Can you work these out from the drawing? Everything is in mm from the part's minimum corner. Coordinates: 2 decimals unless noted, no trailing zeros. Write each loop counter-clockwise with the first axis right and the second up, starting at its lowest first coordinate (ties: lowest second). Pieces come first, ordered by that corner, then holes. Notation, with made-up numbers: (80, 76) -> (90, 76) arc R10 cw to (90, 86) -> close; hole circle Ø1 at (41, 20.5). An arc over 180 degrees is marked (long way). Use a Markdown table: item, result. Add a question column.
Item 1: If we mould it in two halves opening along X, with no side actions, what happens to the marked faces 1 and 2? For each: pulls with the +X half, pulls with the -X half, needs draft (parallel to the pull), parting line crosses it, or undercut.
Item 2: Imagine slicing it at C-C, the plane y = 6.75. Count the separate pieces of the cut face and the enclosed holes in it, and give its area (3 significant figures).
Item 3: Imagine slicing it at B-B, the plane x = 120. Write out the boundary of the cut face in (y, z) (1 decimal).
Item 4: Imagine slicing it at D-D, the plane z = 79. Write out the boundary of the cut face in (x, y) (1 decimal).
Item 5: Imagine slicing it at A-A, the plane z = 15. Write out the boundary of the cut face in (x, y) (1 decimal).
Item 6: If I drill on line 1 along X through (y, z) = (2.25, 79) (1 decimal); line 2 along X through (y, z) = (4, 13.5); line 3 along X through (y, z) = (5.5, 59), over which ranges is the centre line in solid material (lowest first)? Write a range as from..to.
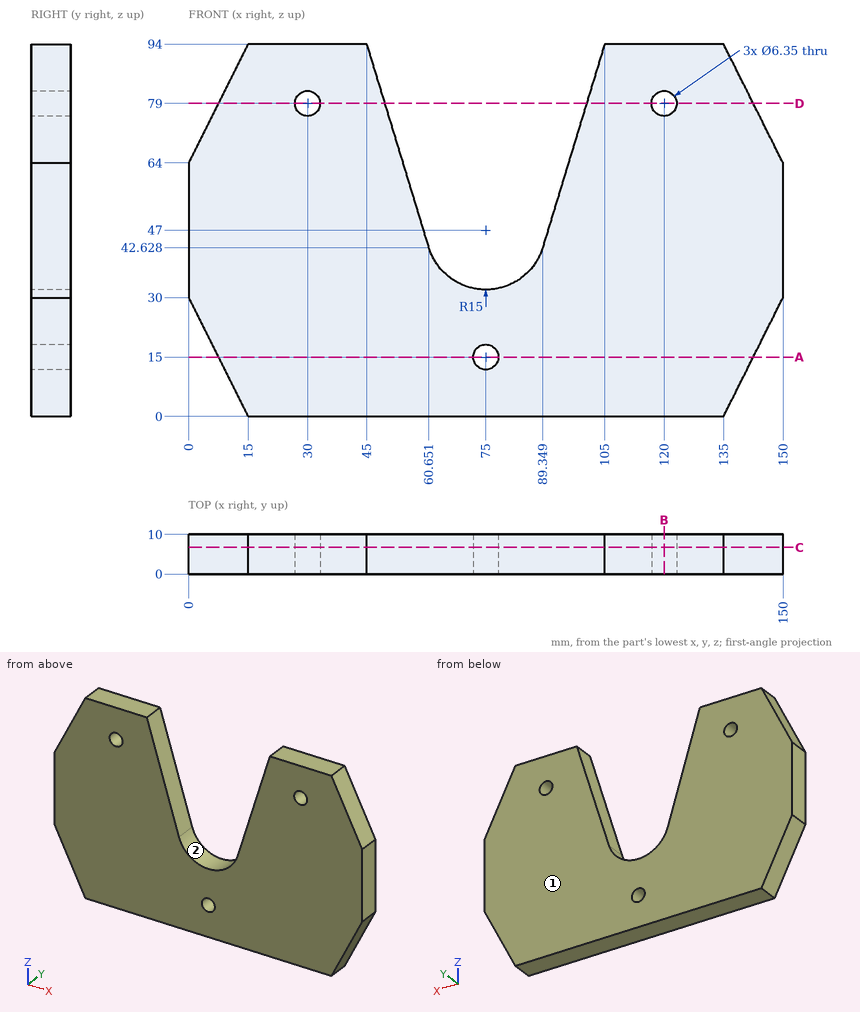
Ans:
| question | item | result |
|---|---|---|
| 1 | face 1 | needs draft |
| 1 | face 2 | undercut |
| 2 | separate pieces | 1 |
| 2 | enclosed holes | 3 |
| 2 | area | 10,600 mm^2 |
| 3 | outline | (0, 0) -> (10, 0) -> (10, 75.8) -> (0, 75.8) -> close; (0, 82.2) -> (10, 82.2) -> (10, 94) -> (0, 94) -> close |
| 4 | outline | (7.5, 0) -> (26.8, 0) -> (26.8, 10) -> (7.5, 10) -> close; (33.2, 0) -> (49.6, 0) -> (49.6, 10) -> (33.2, 10) -> close; (100.4, 0) -> (116.8, 0) -> (116.8, 10) -> (100.4, 10) -> close; (123.2, 0) -> (142.5, 0) -> (142.5, 10) -> (123.2, 10) -> close |
| 5 | outline | (7.5, 0) -> (71.8, 0) -> (71.8, 10) -> (7.5, 10) -> close; (78.2, 0) -> (142.5, 0) -> (142.5, 10) -> (78.2, 10) -> close |
| 6 | line 1 | x = 7.5..26.8, 33.2..49.6, 100.4..116.8, 123.2..142.5 |
| 6 | line 2 | x = 8.25..72.2, 77.8..141.75 |
| 6 | line 3 | x = 0..55.66, 94.34..150 |
